Work out the finished part from the listing and answer in its coordinate system (mm). Face numbers are marked on the shaded views. A direction names the side the tool comes from. Round coordinates to 2 decimals unless told otherwise and drop trailing zeros. Loops run counter-clockwise (first coordinate to the right, second up) from the corner with the lowest first, then second, coordinate; pieces in that order, holes last.
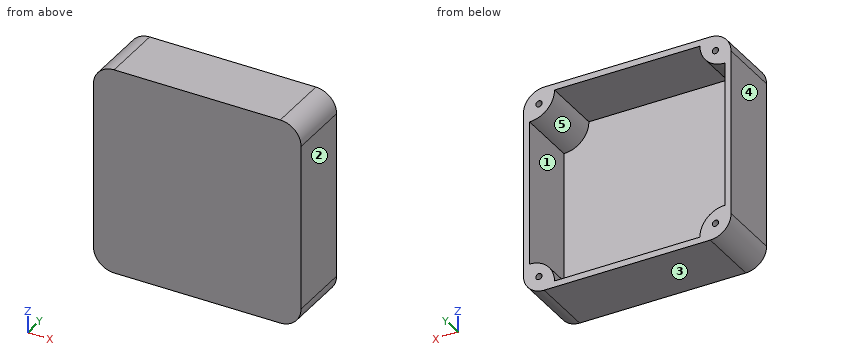
from build123d import *

# Parameters (mm, degrees)
SKIZZE1_R                       = 1.5
AUFSATZ_LINEAR_AUSTRAGEN1_DEPTH = 30
AUFSATZ_LINEAR_AUSTRAGEN2_DEPTH = 1
VERRUNDUNG1_R                   = 10
SKIZZE1_4_R                     = 1.5
AUFSATZ_LINEAR_AUSTRAGEN3_DEPTH = 1
VERRUNDUNG2_R                   = 12


with BuildPart() as part:
    # Skizze1 → Aufsatz-Linear austragen1 (new body)
    with BuildSketch(Plane(origin=(0, 0, 0), x_dir=(1, 0, 0), z_dir=(0, 1, 0))):
        Polygon((-50, 50), (50, 50), (50, -50), (-50, -50), (-50, 35), align=None)
        with Locations(Location((42.5, 42.5, 0), (0, 0, 270))):
            Circle(SKIZZE1_R, mode=Mode.SUBTRACT)
        with Locations(Location((-42.5, 42.5, 0), (0, 0, 270))):
            Circle(SKIZZE1_R, mode=Mode.SUBTRACT)
        with Locations(Location((42.5, -42.5, 0), (0, 0, 270))):
            Circle(SKIZZE1_R, mode=Mode.SUBTRACT)
        with Locations(Location((-42.5, -42.5, 0), (0, 0, 270))):
            Circle(SKIZZE1_R, mode=Mode.SUBTRACT)
        Polygon((-47, -35), (-35, -35), (-35, -47), (35, -47), (35, -35), (47, -35), (47, 35), (35, 35), (35, 47), (-35, 47), (-35, 35), (-47, 35), align=None, mode=Mode.SUBTRACT)
    extrude(amount=AUFSATZ_LINEAR_AUSTRAGEN1_DEPTH)

    # Skizze1<3> → Aufsatz-Linear austragen2 (add)
    with BuildSketch(Plane(origin=(0, 0, 0), x_dir=(1, 0, 0), z_dir=(0, 1, 0))):
        Polygon((-47, -35), (-47, 35), (-35, 35), (-35, 47), (35, 47), (35, 35), (47, 35), (47, -35), (35, -35), (35, -47), (-35, -47), (-35, -35), align=None)
    extrude(amount=AUFSATZ_LINEAR_AUSTRAGEN2_DEPTH)

    # Verrundung1
    verrundung1_edges = [part.edges().sort_by_distance(p)[0] for p in [
        (50, 15, -50),
        (50, 15, 50),
        (-50, 15, 50),
        (-50, 15, -50),
    ]]
    fillet(verrundung1_edges, radius=VERRUNDUNG1_R)

    # Skizze1<4> → Aufsatz-Linear austragen3 (add)
    with BuildSketch(Plane(origin=(0, 0, 0), x_dir=(1, 0, 0), z_dir=(0, 1, 0))):
        with Locations(Location((-42.5, 42.5, 0), (0, 0, 270))):
            Circle(SKIZZE1_4_R)
        with Locations(Location((-42.5, -42.5, 0), (0, 0, 270))):
            Circle(SKIZZE1_4_R)
        with Locations(Location((42.5, -42.5, 0), (0, 0, 270))):
            Circle(SKIZZE1_4_R)
        with Locations(Location((42.5, 42.5, 0), (0, 0, 270))):
            Circle(SKIZZE1_4_R)
    extrude(amount=AUFSATZ_LINEAR_AUSTRAGEN3_DEPTH)

    # Verrundung2
    verrundung2_edges = [part.edges().sort_by_distance(p)[0] for p in [
        (35, 15.5, 35),
        (-35, 15.5, 35),
        (35, 15.5, -35),
        (-35, 15.5, -35),
    ]]
    fillet(verrundung2_edges, radius=VERRUNDUNG2_R - 0.0001)  # a hair under: the kernel refuses the full size


solid = part.part
Item 1: This flat-tipped pin is pushed along its axis until it touches: P1, Ø0.9, axis at x = -42, z = -42, coming from the +Y side. Where does it stop, or does it pass through?
Item 2: Determine the mould class of the marked faces 1, 2 and 3 for opening direction X: pulls with the +X half, pulls with the -X half, needs draft (parallel to the pull), parting line crosses it, or undercut.
Item 3: Section D-D, the plane x = 42.5 is taken. Give the vertices of the cut face in (y, z).
Item 4: For the marked faces 4 and 5, determine the directions among +Z, -Z, +X, -X, +Y, -Y from which every point of the face is accessible in a straight line to the end or side of a thin tool.
Item 5: Section C-C, the plane x = -21 is taken. Give the vertices of the cut face in (y, z), plus the area to 3 significant figures.
Item 6: Section A-A, the plane y = 9.5 is taken. State how many separate pieces and enclosed holes the cut face has, plus the area to 3 significant figures.
Item 7: Straight lines are drawn through the part: line 1 (Z direction, x = 33, y = 12.5); line 2 (X direction, y = 8, z = 42.5). For each, find the intervals that lie inside material, in ascending order.
Item 8: Section B-B, the plane z = 14 is taken. Give the vertices of the cut face in (x, y), plus the area to 3 significant figures.
Answer below:
1. P1: stops at y = 1
2. face 1: undercut
2. face 2: pulls with the +X half
2. face 3: needs draft
3. outline: (0, -49.68) - (30, -49.68) - (30, -44) - (1, -44) - (1, -41) - (30, -41) - (30, -35.88) - (1, -35.88) - (1, 35.88) - (30, 35.88) - (30, 41) - (1, 41) - (1, 44) - (30, 44) - (30, 49.68) - (0, 49.68) - close
4. face 4: +Z, -Z, -X, +Y, -Y
4. face 5: +Y
5. outline: (0, -50) - (30, -50) - (30, -47) - (1, -47) - (1, 47) - (30, 47) - (30, 50) - (0, 50) - close
5. area: 274 mm2
6. separate pieces: 1
6. enclosed holes: 5
6. area: 1,500 mm2
7. line 1: z = -50 to -47, 47 to 50
7. line 2: x = -49.68 to -44, -41 to -35.88, 35.88 to 41, 44 to 49.68
8. outline: (-50, 0) - (50, 0) - (50, 30) - (47, 30) - (47, 1) - (-47, 1) - (-47, 30) - (-50, 30) - close
8. area: 274 mm2
